Part model, mm, in its own coordinate system. Face numbers are marked on the shaded views. A direction names the side the tool comes from. Round coordinates to 2 decimals unless told otherwise and drop trailing zeros. Loops run counter-clockwise (first coordinate to the right, second up) from the corner with the lowest first, then second, coordinate; pieces in that order, holes last. Notation, with made-up numbers: (39.25, 10.5) - (58.25, 10.5) arc R19 cw to (58.25, 32.5) - close; hole circle Ø10 at (-1.75, -36.75). An arc over 180 degrees is marked (long way). Write each question's results on one line, items separated by ' | '. Start each with the question number.
(1) Tool access for the marked faces 1, 2, 3 and 4: list every direction of +Z, -Z, +X, -X, +Y, -Y with a clear straight run to the whole face (end or side of a thin tool).
(2) Cut at B-B, the plane y = 50.5. List the corners of the cut face in (x, z), then the cut area to 3 significant figures.
(3) Cut at C-C, the plane y = 32.5. List the corners of the cut face in (x, z), then the cut area to 3 significant figures.
(4) Flat gauge pins, fed straight in: P1, Ø12, axis at x = 1, y = -17, coming from the +Z side; P2, Ø4, axis at y = 64.58, z = -46.31, coming from the -X side; P3, Ø7.5, axis at x = 0.5, y = -54, coming from the +Z side. Where does each tip first touch, or does it go through?
(5) Cut at D-D, the plane y = 16. List the corners of the cut face in (x, z), then the cut area to 3 significant figures.
(6) Cut at A-A, the plane z = -70. List the corners of the cut face in (x, y).
(7) Mould opens along Y. For the marked faces 5, 6, 7 and 8 say: released by +Y, released by -Y, zero draft, split by the parting line, or undercut.
(8) Drill centre lines: L1, parallel to Y at x = -5.75, z = -80.5; L2, parallel to X at y = -22, z = -60.5; L3, parallel to Y at x = -8, z = -78. Where is each one in solid material? Low to high.
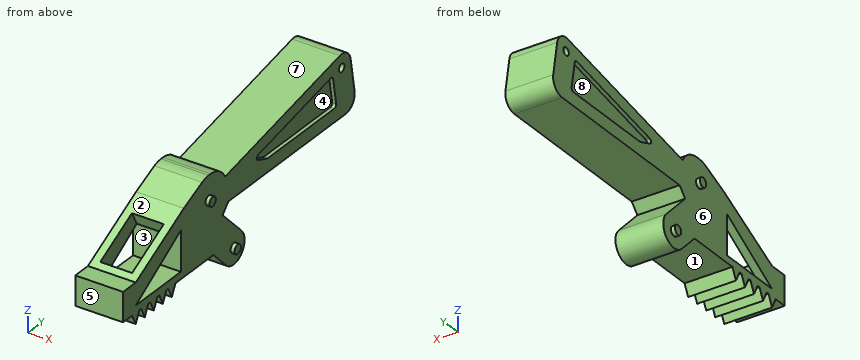
from build123d import *

# Parameters (mm, degrees)
BOSS_EXTRUDE1_DEPTH     = 9
CUT_EXTRUDE1_DEPTH      = 116.769079262
CUT_EXTRUDE1_DEPTH_BACK = 116.769079262
BOSS_EXTRUDE2_DEPTH     = 18
LPATTERN1_COUNT         = 5
LPATTERN1_PITCH         = 5
FILLET1_R               = 9
FILLET2_R               = 5
SKETCH5_R               = 1.5
CUT_EXTRUDE2_DEPTH      = 25
CUT_EXTRUDE3_REACH      = 94.43
SKETCH8_W               = 12
SKETCH8_H               = 19.757506074
SKETCH9_R               = 1.75
BOSS_EXTRUDE3_DEPTH     = 1.5
SKETCH10_R              = 1.75
BOSS_EXTRUDE4_DEPTH     = 1.5
CUT_EXTRUDE5_DEPTH      = 1.5


with BuildPart() as part:
    # Sketch1 → Boss-Extrude1 (new, symmetric)
    with BuildSketch(Plane(origin=(0, 0, 0), x_dir=(0, 0, -1), z_dir=(1, 0, 0))):
        Polygon((64.03845405, 1.736481777), (54.19037652, 0), (40.392944784, 68.626750451), (64.03845405, 72.736481777), align=None)
        with BuildLine():
            Line((79.326468903, -6.518014035), (86.456160579, 0.493939802))
            ThreePointArc((86.456160579, 0.493939802), (86.526803283, 8.978927109), (78.041815975, 9.049569813))
            Line((78.041815975, 9.049569813), (67.436419126, -1.380692322))
            Line((67.436419126, -1.380692322), (64.03845405, 1.736481777))
            Line((64.03845405, 1.736481777), (54.19037652, 0))
            Line((54.19037652, 0), (49.287534486, -0.985718074))
            Line((49.287534486, -0.985718074), (49.287534486, -10.985718074))
            Line((49.287534486, -10.985718074), (54.49039716, -22.899165098))
            Line((54.49039716, -22.899165098), (68.326468903, -49.518014035))
            Line((68.326468903, -49.518014035), (68.326468903, -56.518014035))
            Line((68.326468903, -56.518014035), (79.326468903, -56.518014035))
            Line((79.326468903, -56.518014035), (79.326468903, -6.518014035))
        make_face()
    extrude(amount=BOSS_EXTRUDE1_DEPTH, both=True)

    # Sketch3 → Cut-Extrude1 (cut, two sides: drawn at the far end of the back side and taken through both)
    with BuildSketch(Plane(origin=(9, 0, 0), x_dir=(0, 0, -1), z_dir=(1, 0, 0)).offset(-CUT_EXTRUDE1_DEPTH_BACK)):
        Polygon((76.626468903, -49.518014035), (76.626468903, -24.518014035), (61.626468903, -24.518014035), align=None)
    extrude(amount=CUT_EXTRUDE1_DEPTH + CUT_EXTRUDE1_DEPTH_BACK, mode=Mode.SUBTRACT)

    # Sketch4 → Boss-Extrude2 (add)
    with BuildSketch(Plane(origin=(9, 0, 0), x_dir=(0, 0, -1), z_dir=(1, 0, 0))):
        Polygon((83.326468903, -49.518014035), (79.326468903, -49.518014035), (79.326468903, -51.518014035), align=None)
        Polygon((79.326468903, -47.518014035), (79.326468903, -49.518014035), (83.326468903, -49.518014035), align=None)
    boss_extrude2 = extrude(amount=-BOSS_EXTRUDE2_DEPTH)

    # LPattern1: Boss-Extrude2 ×5
    with Locations(*[(0, i * LPATTERN1_PITCH, 0) for i in range(1, LPATTERN1_COUNT)]):
        add(boss_extrude2)

    # Fillet1
    # the kernel refuses this fillet: 9 mm, written as the material it takes off along each edge
    with BuildSketch(Plane(origin=(-13.698844365, -10.985718074, -49.287534486), x_dir=(0, -0.9164190018423571, -0.4002202057146263), z_dir=(1, 0, 0))) as fillet1_piece_1:
        with BuildLine():
            CenterArc((FILLET1_R * 0.208837527352, FILLET1_R), FILLET1_R, 246.408054679, 23.591945321)
            Line((-FILLET1_R * 0.191382678363, FILLET1_R * 0.0835809981576), (-FILLET1_R * 0.199387082477, FILLET1_R * 0.0652526181208))
            Line((-FILLET1_R * 0.199387082477, FILLET1_R * 0.0652526181208), (-FILLET1_R * 0.00417675054703, -FILLET1_R * 0.02))
            Line((-FILLET1_R * 0.00417675054703, -FILLET1_R * 0.02), (FILLET1_R * 0.208837527352, -FILLET1_R * 0.02))
            Line((FILLET1_R * 0.208837527352, -FILLET1_R * 0.02), (FILLET1_R * 0.208837527352, 0))
        make_face()
    extrude(amount=27.397688731, mode=Mode.SUBTRACT)
    with BuildSketch(Plane(origin=(-26.569004687, -0.985718074, -49.287534486), x_dir=(0, -1, 0), z_dir=(1, 0, 0))) as fillet1_piece_2:
        with BuildLine():
            CenterArc((7.027601875, 9), FILLET1_R, 207.080362773, 62.919637227)
            Line((-0.985718074, 4.902842034), (-1.145984473, 4.820898874))
            ThreePointArc((-1.145984473, 4.820898874), (-0.669327824, 2.415941907), (-0.176468787, -0.03547911))
            Line((-0.176468787, -0.03547911), (0, -0.18))
            Line((0, -0.18), (7.027601875, -0.18))
            Line((7.027601875, -0.18), (7.027601875, 0))
        make_face()
    extrude(amount=53.138009374, mode=Mode.SUBTRACT)

    # Fillet2
    fillet2_edges = [part.edges().sort_by_distance(p)[0] for p in [
        (0, 68.626750451, -40.392944784),
        (0, 72.736481777, -64.03845405),
    ]]
    fillet(fillet2_edges, radius=FILLET2_R)

    # Sketch5 → Cut-Extrude2 (cut)
    with BuildSketch(Plane(origin=(9, 0, 0), x_dir=(0, 0, -1), z_dir=(1, 0, 0))):
        with Locations((46.306671362, 64.579632178)):
            Circle(SKETCH5_R)
    extrude(amount=-CUT_EXTRUDE2_DEPTH, mode=Mode.SUBTRACT)

    # Cut-Extrude3: up to this plane
    cut_extrude3_end = Plane(origin=(-9, -24.518014035, -61.626468903), z_dir=(0, -0.5144957554275262, 0.8574929257125444))
    # Sketch8 → Cut-Extrude3 (cut, up to the surface)
    with BuildSketch(Plane(origin=(0, 17.427872297, -33.529018106), x_dir=(1, 0, 0), z_dir=(0, -0.4612023914177088, 0.8872949645696107)), mode=Mode.PRIVATE) as cut_extrude3_sk1:
        with Locations((0, -62.828168401)):
            Rectangle(SKETCH8_W, SKETCH8_H)
    cut_extrude3_tool1 = split(extrude(cut_extrude3_sk1.sketch, amount=-CUT_EXTRUDE3_REACH, mode=Mode.PRIVATE), bisect_by=cut_extrude3_end, keep=Keep.BOTH, mode=Mode.PRIVATE)
    add(cut_extrude3_tool1.solids().sort_by_distance((0, -38.319245, -62.50552))[0], mode=Mode.SUBTRACT)

    # Sketch9 → Boss-Extrude3 (add)
    with BuildSketch(Plane(origin=(9, 0, 0), x_dir=(0, 0, -1), z_dir=(1, 0, 0))):
        with Locations((82.248988277, 4.771754807)):
            Circle(SKETCH9_R)
    boss_extrude3 = extrude(amount=BOSS_EXTRUDE3_DEPTH)

    # Sketch10 → Boss-Extrude4 (add)
    with BuildSketch(Plane(origin=(9, 0, 0), x_dir=(0, 0, -1), z_dir=(1, 0, 0))):
        with Locations((58.287534486, -9.106180328)):
            Circle(SKETCH10_R)
    boss_extrude4 = extrude(amount=BOSS_EXTRUDE4_DEPTH)

    # Sketch11 → Cut-Extrude5 (cut)
    with BuildSketch(Plane(origin=(9, 0, 0), x_dir=(0, 0, -1), z_dir=(1, 0, 0))):
        with BuildLine():
            Line((59.03845405, 60.528735066), (59.03845405, 23.717958421))
            ThreePointArc((59.03845405, 23.717958421), (59.023347404, 23.544796412), (58.978483887, 23.376866197))
            Line((58.978483887, 23.376866197), (57.101026027, 18.202704248))
            ThreePointArc((57.101026027, 18.202704248), (56.086229397, 17.546595426), (55.180614041, 18.346690305))
            Line((55.180614041, 18.346690305), (47.087922198, 58.598757084))
            ThreePointArc((47.087922198, 58.598757084), (47.2430546, 59.360631218), (47.897065542, 59.781092804))
            Line((47.897065542, 59.781092804), (57.867215244, 61.513964619))
            ThreePointArc((57.867215244, 61.513964619), (58.682178057, 61.293992802), (59.03845405, 60.528735066))
        make_face()
    cut_extrude5 = extrude(amount=-CUT_EXTRUDE5_DEPTH, mode=Mode.SUBTRACT)

    # Mirror1: Cut-Extrude5 across plane
    add(cut_extrude5.mirror(Plane(origin=(0, 0, 0), x_dir=(0, 0, 1), z_dir=(1, 0, 0))), mode=Mode.SUBTRACT)

    # Mirror2: Boss-Extrude3, Boss-Extrude4 across plane
    add(boss_extrude3.mirror(Plane(origin=(0, 0, 0), x_dir=(0, 0, 1), z_dir=(1, 0, 0))))
    add(boss_extrude4.mirror(Plane(origin=(0, 0, 0), x_dir=(0, 0, 1), z_dir=(1, 0, 0))))


solid = part.part
A:
1) face 1: -Z, +X, -X | face 2: +Z, +X, -X, -Y | face 3: +X, -X | face 4: +X
2) outline: (-9, -64.04) - (9, -64.04) - (9, -59.04) - (7.5, -59.04) - (7.5, -48.72) - (9, -48.72) - (9, -44.04) - (-9, -44.04) - (-9, -48.72) - (-7.5, -48.72) - (-7.5, -59.04) - (-9, -59.04) - close | area: 329 mm2
3) outline: (-9, -64.04) - (9, -64.04) - (9, -59.04) - (7.5, -59.04) - (7.5, -52.34) - (9, -52.34) - (9, -47.66) - (-9, -47.66) - (-9, -52.34) - (-7.5, -52.34) - (-7.5, -59.04) - (-9, -59.04) - close | area: 275 mm2
4) P1: z = -49.49 | P2: x = -9 | P3: z = -68.33
5) outline: (-9, -64.04) - (9, -64.04) - (9, -50.97) - (-9, -50.97) - close | area: 235 mm2
6) outline: (-9, -56.52) - (9, -56.52) - (9, -38.47) - (6, -38.47) - (6, -45.56) - (-6, -45.56) - (-6, -38.47) - (-9, -38.47) - close; (-9, -24.52) - (9, -24.52) - (9, 1.14) - (-9, 1.14) - close
7) face 5: released by -Y | face 6: zero draft | face 7: undercut | face 8: undercut
8) L1: -50.93 to -48.1, -45.93 to -43.1, -40.93 to -38.1, -35.93 to -33.1, -30.93 to -28.1, -5.36 to 10.51 | L2: -9 to 9 | L3: -56.52 to 9.01
